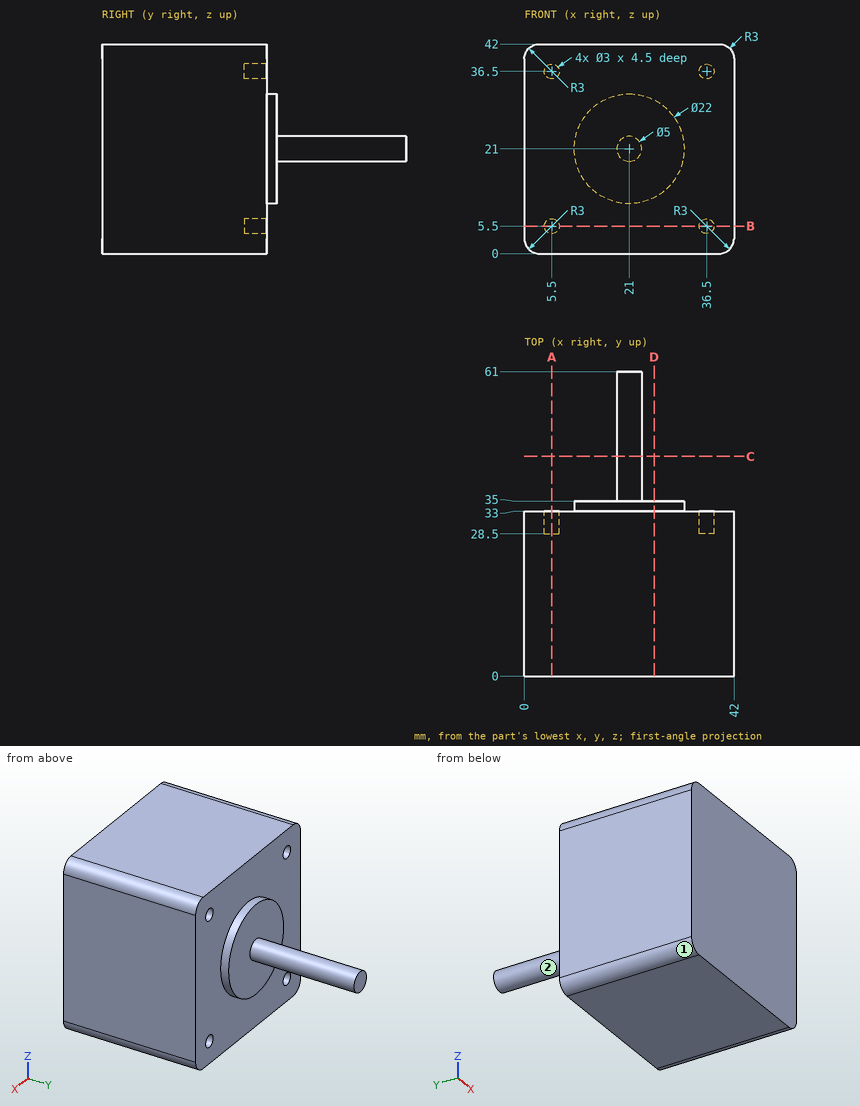
Geometry check sheet. Reference: drawing and pictorial views, mm from the part's lowest x, y, z. A direction names the side the tool comes from. Give positions to 0.01 mm unless a question says otherwise; leave off trailing zeros. Order: outer loops, then holes, each group sorted by start corner. A loop starts at its lowest first (then second) coordinate and runs counter-clockwise, first axis right, second up. Notation, with made-up numbers: (66, 16) - (100, 16) arc R20 ccw to (100, 54) - close; hole circle Ø4 at (23, 60). An arc over 180 degrees is marked (long way). Answer as CSV lines item,"result". Start each with the question number.
Item 1: Section check D-D, the plane x = 26. Record the boundary of the cut face in (y, z), plus the area to 3 significant figures.
Item 2: Section check B-B, the plane z = 5.5. Record the boundary of the cut face in (x, y).
Item 3: Section check A-A, the plane x = 5.5. Record the boundary of the cut face in (y, z).
Item 4: Gauge pin test, flat ends, axial feed: pin 1 (4 mm diameter, centred on x = 36.5, z = 5.5, fed in from +Y); pin 2 (21 mm diameter, centred on x = 10.5, z = 11, fed in from +Y); pin 3 (2.5 mm diameter, centred on x = 5.5, z = 36.5, fed in from +Y). Record the tip position at first contact, or that the pin passes through.
Item 5: Access from +Z, -Z, +X, -X, +Y, -Y to the whole of each face (thin tool, end or side, straight path). Record for the marked faces 1 and 2.
Item 6: Material ranges on L1, parallel to Z at x = 36, y = 31; L2, parallel to Y at x = 23.5, z = 16, recorded low to high.
Item 7: Section check C-C, the plane y = 44. Record the boundary of the cut face in (x, z).
Filled in:
1,outline,"(0, 0) - (33, 0) - (33, 11.2) - (35, 11.2) - (35, 30.8) - (33, 30.8) - (33, 42) - (0, 42) - close"
1,area,"1,430 mm^2"
2,outline,"(0, 0) - (42, 0) - (42, 33) - (38, 33) - (38, 28.5) - (35, 28.5) - (35, 33) - (7, 33) - (7, 28.5) - (4, 28.5) - (4, 33) - (0, 33) - close"
3,outline,"(0, 0) - (33, 0) - (33, 4) - (28.5, 4) - (28.5, 7) - (33, 7) - (33, 35) - (28.5, 35) - (28.5, 38) - (33, 38) - (33, 42) - (0, 42) - close"
4,pin 1,"y = 33"
4,pin 2,"y = 35"
4,pin 3,"y = 28.5"
5,face 1,"-Z, -X, +Y, -Y"
5,face 2,"+Y"
6,L1,"0 to 4.09, 6.91 to 35.09, 37.91 to 42"
6,L2,"0 to 35"
7,outline,"circle Ø5 at (21, 21)"
